```python
from build123d import *

# Parameters (mm, degrees)
SKETCH_2_W                                   = 420
SKETCH_2_H                                   = 420
EXTRUDE_1_DEPTH                              = 3
SKETCH_3_R                                   = 1.6
SKETCH_3_W                                   = 41
SKETCH_3_H                                   = 20.5
SKETCH_3_W_2                                 = 45
SKETCH_3_H_2                                 = 60
CUT_EXTRUDE_1_DEPTH                          = 298
MIRROR_2_AT_THE_SECOND_PLANE_COPY_1_SKET_R   = 1.6
MIRROR_2_AT_THE_SECOND_PLANE_COPY_1_SKET_W   = 41
MIRROR_2_AT_THE_SECOND_PLANE_COPY_1_SKET_H   = 20.5
MIRROR_2_AT_THE_SECOND_PLANE_COPY_1_SKET_W_2 = 45
MIRROR_2_AT_THE_SECOND_PLANE_COPY_1_SKET_H_2 = 60
MIRROR_2_AT_THE_SECOND_PLANE_COPY_1_DEPTH    = 298
SKETCH_7_R                                   = 2.65
CUT_EXTRUDE_5_DEPTH                          = 298
SKETCH_5_R                                   = 2.15
CUT_EXTRUDE_8_DEPTH                          = 298
PATTERN_LINEAR_4_COUNT                       = 5
PATTERN_LINEAR_4_PITCH                       = 50
PATTERN_LINEAR_4_COL_COUNT                   = 5
PATTERN_LINEAR_4_COL_PITCH                   = 50
SKETCH_6_R                                   = 2.15
CUT_EXTRUDE_9_DEPTH                          = 298
PATTERN_LINEAR_5_COUNT                       = 4
PATTERN_LINEAR_5_PITCH                       = 95
SKETCH_9_R                                   = 1.6
CUT_EXTRUDE_7_DEPTH                          = 298
PATTERN_LINEAR_3_COUNT                       = 9
PATTERN_LINEAR_3_PITCH                       = 50
SKETCH_10_R                                  = 27.5
CUT_EXTRUDE_10_DEPTH                         = 298
SKETCH_8_R                                   = 2.15
SKETCH_8_R_2                                 = 1.6
CUT_EXTRUDE_6_DEPTH                          = 298
FILLET_1_R                                   = 10
SKETCH_11_R                                  = 1.6
CUT_EXTRUDE_11_DEPTH                         = 5


with BuildPart() as part:
    # 草图2 → 凸台-拉伸1 (new body)
    with BuildSketch(Plane(origin=(0, 0, 0), x_dir=(1, 0, 0), z_dir=(0, 1, 0))):
        Rectangle(SKETCH_2_W, SKETCH_2_H)
    extrude(amount=EXTRUDE_1_DEPTH)

    # 草图3 → 切除-拉伸1 (cut, through all)
    with BuildSketch(Plane(origin=(0, 0, 0), x_dir=(1, 0, 0), z_dir=(0, 1, 0))):
        with Locations(Location((-204.75, 187.5, 0), (0, 0, 270))):
            Circle(SKETCH_3_R)
        with Locations(Location((-204.75, 177.5, 0), (0, 0, 270))):
            Circle(SKETCH_3_R)
        with Locations(Location((-155.25, 187.5, 0), (0, 0, 270))):
            Circle(SKETCH_3_R)
        with Locations(Location((-155.25, 177.5, 0), (0, 0, 270))):
            Circle(SKETCH_3_R)
        with Locations((-180, 182.5)):
            Rectangle(SKETCH_3_W, SKETCH_3_H)
        with Locations((-187.5, 135)):
            Rectangle(SKETCH_3_W_2, SKETCH_3_H_2)
    cut_extrude_1 = extrude(amount=CUT_EXTRUDE_1_DEPTH, mode=Mode.SUBTRACT)

    # 镜向2: 切除-拉伸1 across plane
    add(cut_extrude_1.mirror(Plane(origin=(0, 0, 0), x_dir=(0, 0, 1), z_dir=(1, 0, 0))), mode=Mode.SUBTRACT)

    # 镜向2 at the second plane: 切除-拉伸1 across plane
    add(cut_extrude_1.mirror(Plane.XY), mode=Mode.SUBTRACT)

    # 镜向2 at the second plane copy 1 sket → 镜向2 at the second plane copy 1 (cut, through all)
    with BuildSketch(Plane(origin=(0, 0, 0), x_dir=(-1, 0, 0), z_dir=(0, 1, 0))):
        with Locations(Location((-204.75, 187.5, 0), (0, 0, 270))):
            Circle(MIRROR_2_AT_THE_SECOND_PLANE_COPY_1_SKET_R)
        with Locations(Location((-204.75, 177.5, 0), (0, 0, 270))):
            Circle(MIRROR_2_AT_THE_SECOND_PLANE_COPY_1_SKET_R)
        with Locations(Location((-155.25, 187.5, 0), (0, 0, 270))):
            Circle(MIRROR_2_AT_THE_SECOND_PLANE_COPY_1_SKET_R)
        with Locations(Location((-155.25, 177.5, 0), (0, 0, 270))):
            Circle(MIRROR_2_AT_THE_SECOND_PLANE_COPY_1_SKET_R)
        with Locations((-180, 182.5)):
            Rectangle(MIRROR_2_AT_THE_SECOND_PLANE_COPY_1_SKET_W, MIRROR_2_AT_THE_SECOND_PLANE_COPY_1_SKET_H)
        with Locations((-187.5, 135)):
            Rectangle(MIRROR_2_AT_THE_SECOND_PLANE_COPY_1_SKET_W_2, MIRROR_2_AT_THE_SECOND_PLANE_COPY_1_SKET_H_2)
    extrude(amount=MIRROR_2_AT_THE_SECOND_PLANE_COPY_1_DEPTH, mode=Mode.SUBTRACT)

    # 草图7 → 切除-拉伸5 (cut, through all)
    with BuildSketch(Plane(origin=(0, 0, 0), x_dir=(1, 0, 0), z_dir=(0, 1, 0))):
        with Locations(Location((-186.25, 95, 0), (0, 0, 270))):
            Circle(SKETCH_7_R)
        with Locations(Location((-186.25, -95, 0), (0, 0, 270))):
            Circle(SKETCH_7_R)
        with Locations(Location((186.25, -95, 0), (0, 0, 270))):
            Circle(SKETCH_7_R)
        with Locations(Location((186.25, 95, 0), (0, 0, 270))):
            Circle(SKETCH_7_R)
    extrude(amount=CUT_EXTRUDE_5_DEPTH, mode=Mode.SUBTRACT)

    # 草图5 → 切除-拉伸8 (cut, through all)
    with BuildSketch(Plane(origin=(0, 0, 0), x_dir=(1, 0, 0), z_dir=(0, 1, 0))):
        with Locations(Location((-65, 0, 0), (0, 0, 270))):
            Circle(SKETCH_5_R)
        with Locations(Location((65, 0, 0), (0, 0, 270))):
            Circle(SKETCH_5_R)
    cut_extrude_8 = extrude(amount=CUT_EXTRUDE_8_DEPTH, mode=Mode.SUBTRACT)

    # 阵列(线性)4: 切除-拉伸8 ×5
    with Locations(*[(0, 0, i * PATTERN_LINEAR_4_PITCH) for i in range(1, PATTERN_LINEAR_4_COUNT)]):
        add(cut_extrude_8, mode=Mode.SUBTRACT)

    # 阵列(线性)4 col: 切除-拉伸8 ×5
    with Locations(*[(0, 0, -i * PATTERN_LINEAR_4_COL_PITCH) for i in range(1, PATTERN_LINEAR_4_COL_COUNT)]):
        add(cut_extrude_8, mode=Mode.SUBTRACT)

    # 草图6 → 切除-拉伸9 (cut, through all)
    with BuildSketch(Plane(origin=(0, 0, 0), x_dir=(1, 0, 0), z_dir=(0, 1, 0))):
        with Locations(Location((-125, -200, 0), (0, 0, 270))):
            Circle(SKETCH_6_R)
        with Locations(Location((125, -200, 0), (0, 0, 270))):
            Circle(SKETCH_6_R)
        with Locations(Location((0, -200, 0), (0, 0, 270))):
            Circle(SKETCH_6_R)
    cut_extrude_9 = extrude(amount=CUT_EXTRUDE_9_DEPTH, mode=Mode.SUBTRACT)

    # 阵列(线性)5: 切除-拉伸9 ×4
    with Locations(*[(0, 0, -i * PATTERN_LINEAR_5_PITCH) for i in range(1, PATTERN_LINEAR_5_COUNT)]):
        add(cut_extrude_9, mode=Mode.SUBTRACT)

    # 草图9 → 切除-拉伸7 (cut, through all)
    with BuildSketch(Plane(origin=(0, 0, 0), x_dir=(1, 0, 0), z_dir=(0, 1, 0))):
        with Locations(Location((-100, -200, 0), (0, 0, 270))):
            Circle(SKETCH_9_R)
        with Locations(Location((-50, -200, 0), (0, 0, 270))):
            Circle(SKETCH_9_R)
        with Locations(Location((50, -200, 0), (0, 0, 270))):
            Circle(SKETCH_9_R)
        with Locations(Location((100, -200, 0), (0, 0, 270))):
            Circle(SKETCH_9_R)
    cut_extrude_7 = extrude(amount=CUT_EXTRUDE_7_DEPTH, mode=Mode.SUBTRACT)

    # 阵列(线性)3: 切除-拉伸7 ×9
    with Locations(*[(0, 0, -i * PATTERN_LINEAR_3_PITCH) for i in range(1, PATTERN_LINEAR_3_COUNT)]):
        add(cut_extrude_7, mode=Mode.SUBTRACT)

    # 草图10 → 切除-拉伸10 (cut, through all)
    with BuildSketch(Plane(origin=(0, 0, 0), x_dir=(1, 0, 0), z_dir=(0, 1, 0))):
        with Locations(Location((-75, 100, 0), (0, 0, 270))):
            Circle(SKETCH_10_R)
        with Locations(Location((75, 100, 0), (0, 0, 270))):
            Circle(SKETCH_10_R)
        with Locations(Location((75, 0, 0), (0, 0, 270))):
            Circle(SKETCH_10_R)
        with Locations(Location((-75, 0, 0), (0, 0, 270))):
            Circle(SKETCH_10_R)
        with Locations(Location((-75, -100, 0), (0, 0, 270))):
            Circle(SKETCH_10_R)
        with Locations(Location((75, -100, 0), (0, 0, 270))):
            Circle(SKETCH_10_R)
    extrude(amount=CUT_EXTRUDE_10_DEPTH, mode=Mode.SUBTRACT)

    # 草图8 → 切除-拉伸6 (cut, through all)
    with BuildSketch(Plane(origin=(0, 0, 0), x_dir=(1, 0, 0), z_dir=(0, 1, 0))):
        with Locations(Location((-200, 80, 0), (0, 0, 270))):
            Circle(SKETCH_8_R)
        with Locations(Location((-200, -80, 0), (0, 0, 270))):
            Circle(SKETCH_8_R)
        with Locations(Location((-200, 0, 0), (0, 0, 270))):
            Circle(SKETCH_8_R)
        with Locations(Location((200, 0, 0), (0, 0, 270))):
            Circle(SKETCH_8_R)
        with Locations(Location((200, 80, 0), (0, 0, 270))):
            Circle(SKETCH_8_R)
        with Locations(Location((200, -80, 0), (0, 0, 270))):
            Circle(SKETCH_8_R)
        with Locations(Location((-167.25, 202.5, 0), (0, 0, 270))):
            Circle(SKETCH_8_R_2)
        with Locations(Location((-181.25, 202.5, 0), (0, 0, 270))):
            Circle(SKETCH_8_R_2)
        with Locations(Location((181.25, 202.5, 0), (0, 0, 270))):
            Circle(SKETCH_8_R_2)
        with Locations(Location((181.25, -202.5, 0), (0, 0, 270))):
            Circle(SKETCH_8_R_2)
        with Locations(Location((-181.25, -202.5, 0), (0, 0, 270))):
            Circle(SKETCH_8_R_2)
        with Locations(Location((167.25, 202.5, 0), (0, 0, 270))):
            Circle(SKETCH_8_R_2)
        with Locations(Location((-167.25, -202.5, 0), (0, 0, 270))):
            Circle(SKETCH_8_R_2)
        with Locations(Location((167.25, -202.5, 0), (0, 0, 270))):
            Circle(SKETCH_8_R_2)
    extrude(amount=CUT_EXTRUDE_6_DEPTH, mode=Mode.SUBTRACT)

    # 圆角1
    fillet_1_edges = [part.edges().sort_by_distance(p)[0] for p in [
        (210, 1.5, -105),
        (210, 1.5, -165),
        (210, 1.5, 165),
        (210, 1.5, 105),
        (-210, 1.5, -165),
        (-210, 1.5, -105),
        (-210, 1.5, 105),
        (-210, 1.5, 165),
        (-210, 1.5, -210),
        (210, 1.5, -210),
        (210, 1.5, 210),
        (-210, 1.5, 210),
    ]]
    fillet(fillet_1_edges, radius=FILLET_1_R)

    # 草图11 → 切除-拉伸11 (cut)
    with BuildSketch(Plane(origin=(0, 3, 0), x_dir=(1, 0, 0), z_dir=(0, 1, 0))):
        with Locations(Location((-20, 202.5, 0), (0, 0, 270))):
            Circle(SKETCH_11_R)
        with Locations(Location((20, 202.5, 0), (0, 0, 270))):
            Circle(SKETCH_11_R)
        with Locations(Location((-20, 192.5, 0), (0, 0, 270))):
            Circle(SKETCH_11_R)
        with Locations(Location((20, 192.5, 0), (0, 0, 270))):
            Circle(SKETCH_11_R)
    extrude(amount=-CUT_EXTRUDE_11_DEPTH, mode=Mode.SUBTRACT)


solid = part.part
```
Geometry check sheet. Reference: the model listing, model coordinates, mm. A direction names the side the tool comes from. Round coordinates to 2 decimals unless told otherwise and drop trailing zeros. Write each loop counter-clockwise with the first axis right and the second up, starting at its lowest first coordinate (ties: lowest second). Pieces come first, ordered by that corner, then holes. Notation, with made-up numbers: (-39, 48.5) -> (13, 48.5) arc R22 ccw to (13, 77.5) -> close; hole circle Ø6 at (16.25, 37). An arc over 180 degrees is marked (long way). Put each result on its own line as item: value.
1) Cross-section at B-B, the plane y = 0.6. Give the number of separate pieces and of enclosed holes in the cut face, plus the area to 3 significant figures.
Recorded:
separate pieces: 1
enclosed holes: 96
area: 147,000 mm2
2) Depth check by flat-ended pin: P1, Ø2.5, axis at x = 0, z = 10, coming from the -Y side. Enter the tip coordinate at first touch or a pass-through.
Recorded:
P1: passes through
3) Cross-section at A-A, the plane z = 118. Enter the section's corners in (x, y), plus the area to 3 significant figures.
Recorded:
outline: (-165, 0) -> (-95.79, 0) -> (-95.79, 3) -> (-165, 3) -> close; (-54.21, 0) -> (54.21, 0) -> (54.21, 3) -> (-54.21, 3) -> close; (95.79, 0) -> (165, 0) -> (165, 3) -> (95.79, 3) -> close
area: 741 mm2
4) Access from +Z, -Z, +X, -X, +Y, -Y to the whole of each face (thin tool, end or side, straight path). Record for faces 1 (the face through (206.99, 1.52, -167.85)), 2 (the face through (-3, 3, -3)), 3 (the face through (-206.99, 1.52, 102.15)).
Recorded:
face 1: +X, +Y, -Y
face 2: +Z, -Z, +X, -X, +Y
face 3: -X, +Y, -Y
5) Thickness scan on probe 1 along X at (y, z) = (2.2, -185); probe 2 along Z at (x, y) = (-183.5, 1.45); probe 3 along X at (y, z) = (2.25, 0). Record the ranges inside material, lowest first. Write a range as from..to.
Recorded:
probe 1: x = -210..-200.5, -159.5..159.5, 200.5..210
probe 2: z = -210..-192.75, -172.25..-165, -105..105, 165..172.25, 192.75..210
probe 3: x = -210..-202.15, -197.85..-102.5, -47.5..47.5, 102.5..197.85, 202.15..210
